The model under review builds one solid part; all positions refer to its coordinate system, in mm. A direction names the side the tool comes from. Coordinates: 2 decimals unless noted, no trailing zeros. Write each loop counter-clockwise with the first axis right and the second up, starting at its lowest first coordinate (ties: lowest second). Pieces come first, ordered by that corner, then holes. Notation, with made-up numbers: M 43.5,17.25 L 86.5,17.25 A19 cw 86.5,22.25 Z; hole C -12,85.25 d7. An arc over 180 degrees is marked long. Answer as a JSON object with one key per item and string values.
```python
from build123d import *

# Parameters (mm, degrees)
CROQUIS1_W              = 97.7
CROQUIS1_H              = 85
CROQUIS1_R              = 3
CROQUIS1_R_2            = 30
SALIENTE_EXTRUIR1_DEPTH = 10
CROQUIS2_R              = 5
SALIENTE_EXTRUIR2_DEPTH = 350
CROQUIS3_W              = 97.7
CROQUIS3_H              = 85
SALIENTE_EXTRUIR3_DEPTH = 20


with BuildPart() as part:
    # Croquis1 → Saliente-Extruir1 (new body)
    with BuildSketch(Plane.XY):
        Rectangle(CROQUIS1_W, CROQUIS1_H)
        with Locations((-34.85, 36.5)):
            Circle(CROQUIS1_R, mode=Mode.SUBTRACT)
        Circle(CROQUIS1_R_2, mode=Mode.SUBTRACT)
        with Locations(Location((34.85, 36.5, 0), (0, 0, 180))):
            Circle(CROQUIS1_R, mode=Mode.SUBTRACT)
        with Locations((34.85, -36.5)):
            Circle(CROQUIS1_R, mode=Mode.SUBTRACT)
        with Locations(Location((-34.85, -36.5, 0), (0, 0, 180))):
            Circle(CROQUIS1_R, mode=Mode.SUBTRACT)
    extrude(amount=SALIENTE_EXTRUIR1_DEPTH)

    # Croquis2 → Saliente-Extruir2 (add)
    with BuildSketch(Plane.XY.offset(10)):
        with Locations((-40, 0)):
            Circle(CROQUIS2_R)
        with Locations(Location((40, 0, 0), (0, 0, 180))):
            Circle(CROQUIS2_R)
    extrude(amount=SALIENTE_EXTRUIR2_DEPTH)

    # Croquis3 → Saliente-Extruir3 (add)
    with BuildSketch(Plane.XY.offset(360)):
        Rectangle(CROQUIS3_W, CROQUIS3_H)
    extrude(amount=SALIENTE_EXTRUIR3_DEPTH)


solid = part.part
```
(1) For faces 1 (the face through (-1, 42.5, 370)), 2 (the face through (45, 0, 183)), 3 (the face through (-29.97, 1.32, 4.93)), list the 3-axis set-ups (+Z, -Z, +X, -X, +Y, -Y) from which the entire face can be reached by the end or side of a thin tool; tool diameter is ignored.
Results list:
{"face 1": "+Z, -Z, +X, -X, +Y", "face 2": "none", "face 3": "-Z"}
(2) For pin 1 Ø5 at (x, y) = (-34.85, -36.5) entering from -Z; pin 2 Ø8 at (x, z) = (32.5, 292.5) entering from +Y, all flat-tipped, find the tip position at first contact; note any pin that passes through.
Results list:
{"pin 1": "z = 360", "pin 2": "y = 3.57"}
(3) Add section A-A on x = 0. Give the boundary of the cut face in (y, z).
Results list:
{"outline": "M -42.5,0 L -30,0 L -30,10 L -42.5,10 Z; M -42.5,360 L 42.5,360 L 42.5,380 L -42.5,380 Z; M 30,0 L 42.5,0 L 42.5,10 L 30,10 Z"}
(4) Draft analysis for pull direction X (two halves, no side actions). For faces 4 (the face through (48.85, -1, 370)), 5 (the face through (-45, 0, 183)), 6 (the face through (-48.85, -1, 370)), state which applies: released by +X, released by -X, zero draft, split by the parting line, or undercut.
Results list:
{"face 4": "released by +X", "face 5": "undercut", "face 6": "released by -X"}
(5) Wall thickness on line 1 along Y through (x, z) = (-34.85, 6.5); line 2 along Z through (x, y) = (7.5, -39); line 3 along Y through (x, z) = (0, 3): over which ranges is each line inside the solid? List them lowest first. Write a range as from..to.
Results list:
{"line 1": "-42.5..-39.5, -33.5..33.5, 39.5..42.5", "line 2": "0..10, 360..380", "line 3": "-42.5..-30, 30..42.5"}
(6) Add section D-D on x = -41.5. Give the boundary of the cut face in (y, z).
Results list:
{"outline": "M -42.5,0 L 42.5,0 L 42.5,10 L 4.77,10 L 4.77,360 L 42.5,360 L 42.5,380 L -42.5,380 L -42.5,360 L -4.77,360 L -4.77,10 L -42.5,10 Z"}
(7) Add section C-C on x = 20.5. Give the boundary of the cut face in (y, z).
Results list:
{"outline": "M -42.5,0 L -21.9,0 L -21.9,10 L -42.5,10 Z; M -42.5,360 L 42.5,360 L 42.5,380 L -42.5,380 Z; M 21.9,0 L 42.5,0 L 42.5,10 L 21.9,10 Z"}
(8) Add section B-B on z = 355.5. Give the boundary of the cut face in (x, y), and give its area (3 significant figures).
Results list:
{"outline": "C -40,0 d10; C 40,0 d10", "area": "157 mm²"}
